from build123d import *

# Parameters (mm, degrees)
SKETCH3_W           = 113
SKETCH3_H           = 43
BOSS_EXTRUDE1_DEPTH = 10
SKETCH5_R           = 7.5
BOSS_EXTRUDE3_DEPTH = 8
CUT_EXTRUDE5_DEPTH  = 133.252986734


with BuildPart() as part:
    # Sketch3 → Boss-Extrude1 (new, symmetric)
    with BuildSketch(Plane(origin=(0, 0, 0), x_dir=(1, 0, 0), z_dir=(0, 1, 0))):
        Rectangle(SKETCH3_W, SKETCH3_H)
    extrude(amount=BOSS_EXTRUDE1_DEPTH, both=True)

    # Sketch5 → Boss-Extrude3 (add)
    with BuildSketch(Plane.XY.offset(21.5)):
        with BuildLine():
            Line((56.5, 0), (-56.5, 0))
            Line((-56.5, 0), (-56.5, 18))
            Line((-56.5, 18), (-62.5, 18))
            Line((-62.5, 18), (-62.5, 23.091525958))
            ThreePointArc((-62.5, 23.091525958), (-62.119397663, 25.00494312), (-61.035533906, 26.627059864))
            Line((-61.035533906, 26.627059864), (-38.081296885, 49.581296885))
            ThreePointArc((-38.081296885, 49.581296885), (-31.81001697, 53.139493432), (-24.601457677, 52.977051582))
            Line((-24.601457677, 52.977051582), (58.938576503, 27.880105878))
            ThreePointArc((58.938576503, 27.880105878), (61.512037046, 26.075409123), (62.5, 23.091525958))
            Line((62.5, 23.091525958), (62.5, 18))
            Line((62.5, 18), (56.5, 18))
            Line((56.5, 18), (56.5, 0))
        make_face()
        with Locations((-28.5, 40)):
            Circle(SKETCH5_R, mode=Mode.SUBTRACT)
    boss_extrude3 = extrude(amount=-BOSS_EXTRUDE3_DEPTH)

    # Mirror1: Boss-Extrude3 across plane
    add(boss_extrude3.mirror(Plane.XY))

    # Sketch4 → Cut-Extrude5 (cut, through all)
    with BuildSketch(Plane(origin=(56.5, 0, 0), x_dir=(0, 0, -1), z_dir=(1, 0, 0))):
        with BuildLine():
            ThreePointArc((21.5, -1.451111641), (0, 0), (-21.5, -1.451111641))
            Line((-21.5, -1.451111641), (-21.5, -10))
            Line((-21.5, -10), (21.5, -10))
            Line((21.5, -10), (21.5, -1.451111641))
        make_face()
        with BuildLine():
            Line((-21.5, -10), (-21.5, -1.451111641))
            ThreePointArc((-21.5, -1.451111641), (-105.261578936, -280.498962651), (160, -160))
            ThreePointArc((160, -160), (120.498962651, -54.738421064), (21.5, -1.451111641))
            Line((21.5, -1.451111641), (21.5, -10))
            Line((21.5, -10), (-21.5, -10))
        make_face()
    extrude(amount=-CUT_EXTRUDE5_DEPTH, mode=Mode.SUBTRACT)


solid = part.part
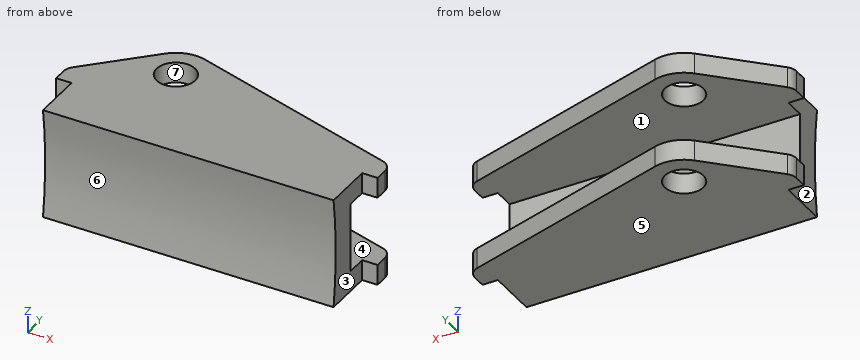
Can you work these out from the model? Positions are in its coordinate system, mm. Face numbers are marked on the shaded views. A direction names the side the tool comes from. Round coordinates to 2 decimals unless told otherwise and drop trailing zeros. Write each loop counter-clockwise with the first axis right and the second up, starting at its lowest first coordinate (ties: lowest second). Pieces come first, ordered by that corner, then holes. Notation, with made-up numbers: (31, 73) -> (46, 73) arc R27 ccw to (46, 104) -> close; hole circle Ø5 at (74.5, -40). An arc over 180 degrees is marked (long way). One line per question, with ' | ' between items. Start each with the question number.
1) If we mould it in two halves opening along Z, with no side actions, what happens to the marked faces 4, 5, 6 and 7? For each: released by +Z, released by -Z, zero draft, split by the parting line, or undercut.
2) Suppose I cut it at A-A on x = -28.5. Write out the boundary of the cut face in (y, z), then the cut area to 3 significant figures.
3) Suppose I cut it at B-B on y = 44.5. Write out the boundary of the cut face in (x, z).
4) I need wall thicknesses on line 1 (Z direction, x = -3, y = 43); line 2 (Y direction, x = -28, z = -1); line 3 (X direction, y = 6.5, z = -19). Which ranges of each line are inside material? Lowest first, please. Write a range as [from, to].
5) I'm going to push flat-ended pins straight in: P1, Ø6, axis at x = 37.5, z = -4.5, coming from the +Y side; P2, Ø1.5, axis at x = -26, z = 12.5, coming from the -Y side; P3, Ø3, axis at y = 27.5, z = 15, coming from the +X side. Where does each tip first touch, or does it pass through?
6) On a 3-axis mill with a long thin cutter (end or side, diameter ignored), from which of +Z, -Z, +X, -X, +Y, -Y can I reach the whole of each face in a straight line? I mean the marked faces 1, 2 and 3. Say none if no direction works.
7) Suppose I cut it at C-C on z = 17.5. Write out the boundary of the cut face in (x, y), then the cut area to 3 significant figures.
8) Suppose I cut it at D-D on x = 22.5. Write out the boundary of the cut face in (y, z), then the cut area to 3 significant figures.
Return value:
1) face 4: undercut | face 5: released by -Z | face 6: undercut | face 7: zero draft
2) outline: (-1.45, -21.5) -> (32.5, -21.5) -> (32.5, -13.5) -> (10, -13.5) -> (10, 13.5) -> (32.5, 13.5) -> (32.5, 21.5) -> (-1.45, 21.5) arc R160 cw to start; (47.5, -21.5) -> (53.55, -21.5) -> (53.55, -13.5) -> (47.5, -13.5) -> close; (47.5, 13.5) -> (53.55, 13.5) -> (53.55, 21.5) -> (47.5, 21.5) -> close | area: 908 mm2
3) outline: (-43.16, -21.5) -> (-34.5, -21.5) -> (-34.5, -13.5) -> (-43.16, -13.5) -> close; (-43.16, 13.5) -> (-34.5, 13.5) -> (-34.5, 21.5) -> (-43.16, 21.5) -> close; (-22.5, -21.5) -> (3.62, -21.5) -> (3.62, -13.5) -> (-22.5, -13.5) -> close; (-22.5, 13.5) -> (3.62, 13.5) -> (3.62, 21.5) -> (-22.5, 21.5) -> close
4) line 1: z = [-21.5, -13.5], [13.5, 21.5] | line 2: y = [0, 10] | line 3: x = [-56.5, 56.5]
5) P1: stops at y = 10 | P2: stops at y = -0.55 | P3: stops at x = 61.57
6) face 1: +X, -X, +Y | face 2: +Z, -Z, -X, -Y | face 3: +Z, -Z, +X, -Y
7) outline: (-62.5, 18) -> (-56.5, 18) -> (-56.5, -0.96) -> (56.5, -0.96) -> (56.5, 18) -> (62.5, 18) -> (62.5, 23.09) arc R5 ccw to (58.94, 27.88) -> (-24.6, 52.98) arc R13.55 ccw to (-38.08, 49.58) -> (-61.04, 26.63) arc R5 ccw to (-62.5, 23.09) -> close; hole circle Ø15 at (-28.5, 40) | area: 4,810 mm2
8) outline: (-1.45, -21.5) -> (38.83, -21.5) -> (38.83, -13.5) -> (10, -13.5) -> (10, 13.5) -> (38.83, 13.5) -> (38.83, 21.5) -> (-1.45, 21.5) arc R160 cw to start | area: 912 mm2
